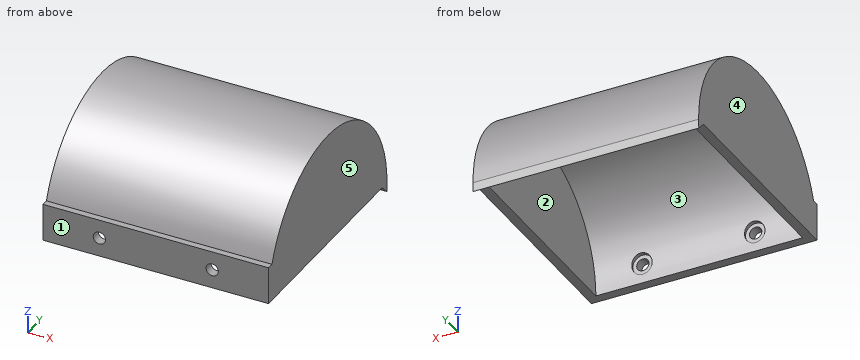
from build123d import *

# Parameters (mm, degrees)
BOSS_EXTRUDE1_DEPTH = 38.1
SHELL1_T            = -3.175
SKETCH7_W           = 76.2
SKETCH7_H           = 3.175
BOSS_EXTRUDE2_DEPTH = 12.7
BOSS_EXTRUDE3_DEPTH = 76.2
CUT_EXTRUDE3_REACH  = 78.2
SKETCH10_R          = 2.0828
CUT_EXTRUDE4_REACH  = 81.375
CUT_EXTRUDE4_START  = -3.175
SKETCH11_R          = 3.429


with BuildPart() as part:
    # Sketch2 → Boss-Extrude1 (new body, symmetric)
    with BuildSketch(Plane(origin=(0, 0, 0), x_dir=(0, 0, -1), z_dir=(1, 0, 0))):
        with BuildLine():
            Line((0, 0), (0, 38.1))
            Line((0, 38.1), (0, 76.2))
            ThreePointArc((0, 76.2), (-38.1, 38.1), (0, 0))
        make_face()
    extrude(amount=BOSS_EXTRUDE1_DEPTH, both=True)

    # Shell1
    shell1_openings = [part.faces().sort_by_distance(p)[0] for p in [
        (0, 38.1, 0),
    ]]
    offset(amount=SHELL1_T, openings=shell1_openings)

    # Sketch7 → Boss-Extrude2 (add)
    with BuildSketch(Plane(origin=(0, 0, 0), x_dir=(1, 0, 0), z_dir=(0, 0, -1))):
        with Locations((0, -1.5875)):
            Rectangle(SKETCH7_W, SKETCH7_H)
    extrude(amount=-BOSS_EXTRUDE2_DEPTH)

    # Sketch8 → Boss-Extrude3 (add)
    with BuildSketch(Plane(origin=(38.1, 0, 0), x_dir=(0, 0, -1), z_dir=(1, 0, 0))):
        Polygon((0, 73.025), (0, 76.2), (3.052521174, 76.077521174), align=None)
    extrude(amount=-BOSS_EXTRUDE3_DEPTH)

    # Sketch10 → Cut-Extrude3 (cut, up to next)
    with BuildSketch(Plane.XZ, mode=Mode.PRIVATE) as cut_extrude3_sk1:
        with Locations((19.05, 6.35)):
            Circle(SKETCH10_R)
    cut_extrude3_tool1 = extrude(cut_extrude3_sk1.sketch, amount=-CUT_EXTRUDE3_REACH, mode=Mode.PRIVATE) & part.part
    add(cut_extrude3_tool1.solids().sort_by_distance((19.05, 0, 6.35))[0], mode=Mode.SUBTRACT)
    # Sketch10 → Cut-Extrude3 (cut, up to next)
    with BuildSketch(Plane.XZ, mode=Mode.PRIVATE) as cut_extrude3_sk2:
        with Locations((-19.05, 6.35)):
            Circle(SKETCH10_R)
    cut_extrude3_tool2 = extrude(cut_extrude3_sk2.sketch, amount=-CUT_EXTRUDE3_REACH, mode=Mode.PRIVATE) & part.part
    add(cut_extrude3_tool2.solids().sort_by_distance((-19.05, 0, 6.35))[0], mode=Mode.SUBTRACT)

    # Sketch11 → Cut-Extrude4 (cut, up to next)
    with BuildSketch(Plane.XZ.offset(CUT_EXTRUDE4_START), mode=Mode.PRIVATE) as cut_extrude4_sk1:
        with Locations((19.05, 6.35)):
            Circle(SKETCH11_R)
    cut_extrude4_tool1 = extrude(cut_extrude4_sk1.sketch, amount=-CUT_EXTRUDE4_REACH, mode=Mode.PRIVATE) & part.part
    add(cut_extrude4_tool1.solids().sort_by_distance((19.05, 3.175, 6.35))[0], mode=Mode.SUBTRACT)
    # Sketch11 → Cut-Extrude4 (cut, up to next)
    with BuildSketch(Plane.XZ.offset(CUT_EXTRUDE4_START), mode=Mode.PRIVATE) as cut_extrude4_sk2:
        with Locations((-19.05, 6.35)):
            Circle(SKETCH11_R)
    cut_extrude4_tool2 = extrude(cut_extrude4_sk2.sketch, amount=-CUT_EXTRUDE4_REACH, mode=Mode.PRIVATE) & part.part
    add(cut_extrude4_tool2.solids().sort_by_distance((-19.05, 3.175, 6.35))[0], mode=Mode.SUBTRACT)


solid = part.part
For this review, take the finished solid that the model builds, in its own axes (mm). Face numbers are marked on the shaded views. A direction names the side the tool comes from. Round coordinates to 2 decimals unless told otherwise and drop trailing zeros. Write each loop counter-clockwise with the first axis right and the second up, starting at its lowest first coordinate (ties: lowest second). Pieces come first, ordered by that corner, then holes. Notation, with made-up numbers: (27, 39) -> (84, 39) arc R17 cw to (84, 65) -> close; hole circle Ø7 at (5, 37). An arc over 180 degrees is marked (long way). Use CSV: the item, a comma, the result in double quotes.
(1) Consider section C-C, the plane x = 31. Give the boundary of the cut face in (y, z) (3 decimals).
Computed values:
outline,"(0, 0) -> (3.175, 0) arc R34.925 cw to (73.025, 0) -> (76.078, -3.053) -> (76.2, 0) arc R38.1 ccw to (2.179, 12.7) -> (0, 12.7) -> close"
(2) Consider section B-B, the plane z = 6.35. Give the boundary of the cut face in (x, y) (3 decimals).
Computed values:
outline,"(-38.1, 0) -> (-21.133, 0) -> (-21.133, 3.175) -> (-22.479, 3.175) -> (-22.479, 3.757) -> (-34.925, 3.757) -> (-34.925, 72.443) -> (34.925, 72.443) -> (34.925, 3.757) -> (22.479, 3.757) -> (22.479, 3.175) -> (21.133, 3.175) -> (21.133, 0) -> (38.1, 0) -> (38.1, 75.667) -> (-38.1, 75.667) -> close; (-16.967, 0) -> (16.967, 0) -> (16.967, 3.175) -> (15.621, 3.175) -> (15.621, 3.757) -> (-15.621, 3.757) -> (-15.621, 3.175) -> (-16.967, 3.175) -> close"
(3) Draft analysis for pull direction X (two halves, no side actions). For the marked faces 3, 4 and 5, state which applies: +X half, -X half, draft (parallel to the pull), parting line (faces both ways), or undercut.
Computed values:
face 3,"undercut"
face 4,"-X half"
face 5,"+X half"
(4) To check wall thickness, follow L1, parallel to X at y = 47.5, z = 26.5 (3 decimals); L2, parallel to X at y = 3, z = 6; L3, parallel to Z at x = -19.05, y = 2. State the ranges of each line that lie inside material, in increasing order. Write a range as [from, to].
Computed values:
L1,"[-38.1, -34.925], [34.925, 38.1]"
L2,"[-38.1, -21.1], [-17, 17], [21.1, 38.1]"
L3,"[0, 4.27], [8.43, 12.7]"
(5) Consider section D-D, the plane z = 20.5. Give the boundary of the cut face in (x, y) (3 decimals), plus the area to 3 significant figures.
Computed values:
outline,"(-38.1, 5.985) -> (38.1, 5.985) -> (38.1, 70.215) -> (-38.1, 70.215) -> close; hole (-34.925, 9.824) -> (34.925, 9.824) -> (34.925, 66.376) -> (-34.925, 66.376) -> close"
area,"944 mm²"
(6) Clearance check with flat-ended pins moving along their axes: P1, Ø2, axis at x = 19, z = 5.5, coming from the -Y side; P2, Ø4, axis at x = 5, z = 25.5, coming from the -Y side; P3, Ø2, axis at x = -19.5, z = 6.5, coming from the +Y side. State where each tip first meets the part, or that it passes through.
Computed values:
P1,"y = 72.41"
P2,"y = 8.11"
P3,"y = 75.8"
(7) For the marked faces 1 and 2, list the 3-axis set-ups (+Z, -Z, +X, -X, +Y, -Y) from which the entire face can be reached by the end or side of a thin tool; tool diameter is ignored.
Computed values:
face 1,"+Z, -Z, +X, -X, -Y"
face 2,"-Z"
(8) Consider section A-A, the plane y = 38.1. Give the boundary of the cut face in (x, z) (3 decimals).
Computed values:
outline,"(-38.1, 0) -> (-34.925, 0) -> (-34.925, 34.925) -> (34.925, 34.925) -> (34.925, 0) -> (38.1, 0) -> (38.1, 38.1) -> (-38.1, 38.1) -> close"
